Answer from the drawing. Dimensions are ordinates in mm from the lowest x, y and z of the part. A direction names the side the tool comes from. Give positions to 0.01 mm unless a question says otherwise; leave off trailing zeros. Write each loop counter-clockwise with the first axis right and the second up, starting at its lowest first coordinate (ties: lowest second). Pieces come first, ordered by that corner, then holes. Notation, with made-up numbers: M 80,-5 L 124,-5 A18 cw 124,23 Z; hole C 82.25,37.5 d8. An arc over 180 degrees is marked long. Put each result on its own line as item: value.
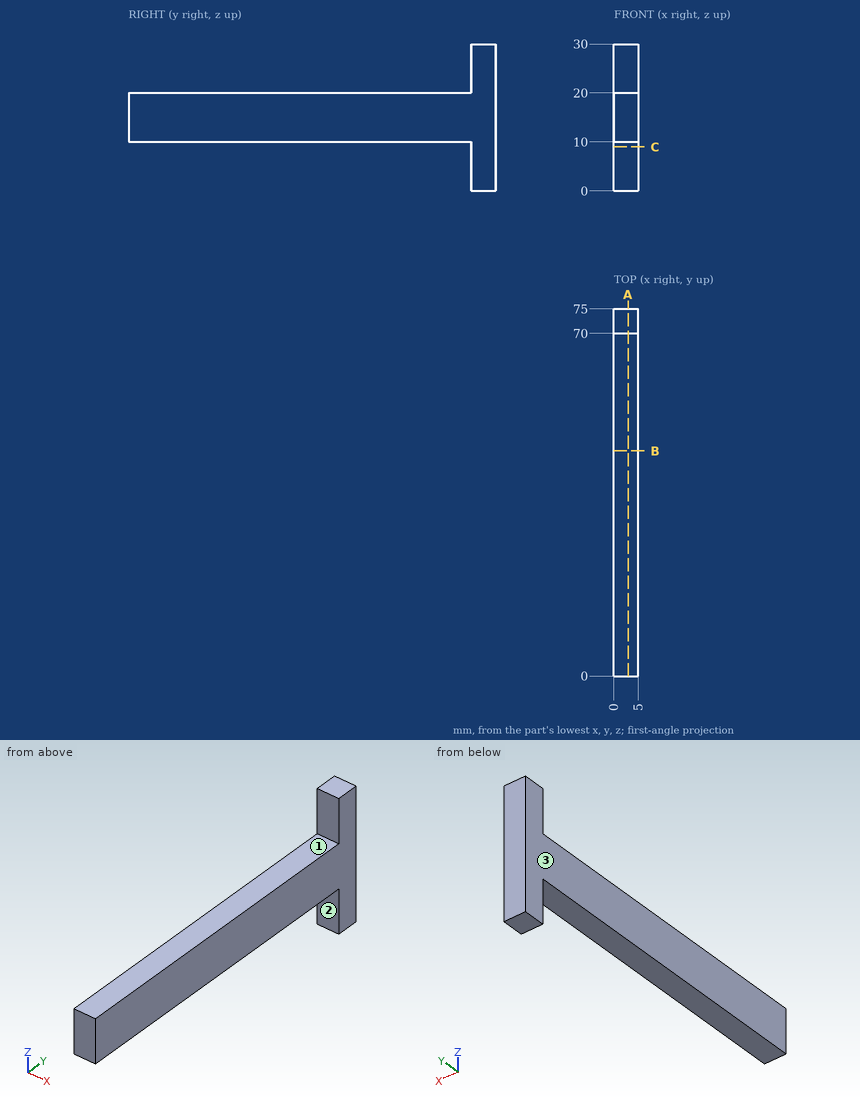
(1) Section B-B on y = 46 is taken. Determine the outline of the cut face in (x, z).
Result:
outline: M 0,10 L 5,10 L 5,20 L 0,20 Z
(2) Which of the six approach directions +Z, -Z, +X, -X, +Y, -Y give full straight-line access (tool end or side, diameter ignored) to the marked faces 1, 2 and 3?
Result:
face 1: +Z, +X, -X, -Y
face 2: -Z, +X, -X, -Y
face 3: +Z, -Z, -X, +Y, -Y
(3) Section A-A on x = 2.9 is taken. Determine the outline of the cut face in (y, z), and give its area (3 significant figures).
Result:
outline: M 0,10 L 70,10 L 70,0 L 75,0 L 75,30 L 70,30 L 70,20 L 0,20 Z
area: 850 mm²
(4) Given pin 1 Ø1 at (x, z) = (3.5, 4) entering from -Y; pin 2 Ø2.5 at (x, y) = (2.5, 51) entering from +Z; pin 3 Ø12 at (y, z) = (21.5, 15.5) entering from -X; pin 4 Ø1.5 at (x, y) = (3, 27) entering from -Z, each flat-ended and moving along its own axis, determine where each tip first touches the part or whether it passes through.
Result:
pin 1: stops at y = 70
pin 2: stops at z = 20
pin 3: stops at x = 0
pin 4: stops at z = 10
(5) Section C-C on z = 9 is taken. Determine the outline of the cut face in (x, y).
Result:
outline: M 0,70 L 5,70 L 5,75 L 0,75 Z
(6) Straight lines are drawn through the part: line 1 along Y through (x, z) = (0.45, 27.75); line 2 along Z through (x, y) = (0.65, 43). For each, find the intervals that lie inside material, in ascending order. Write a range as from..to.
Result:
line 1: y = 70..75
line 2: z = 10..20
